Build history of the part. All positions in model axes, mm. Give positions to 0.01 mm unless a question says otherwise; leave off trailing zeros. Order: outer loops, then holes, each group sorted by start corner. A loop starts at its lowest first (then second) coordinate and runs counter-clockwise, first axis right, second up. Notation, with made-up numbers: M 34.25,-19.75 L 52.25,-19.75 A8 ccw 52.25,-11.75 Z; hole C 51.25,-8.5 d6. An arc over 180 degrees is marked long. Use CSV: the item, a comma, the result in double quotes. Start each with the question number.
Item 1: Wall check: line 1 along X through (y, z) = (29.5, -5); line 2 along Y through (x, z) = (41, -1.5); line 3 along X through (y, z) = (-29, -12.5). Give the ranges that are in metal, low to high.
Item 2: Band-saw the part on A-A on x = 0. Write the cut outline in (y, z), plus the area to 3 significant figures.
Item 3: Band-saw the part on D-D on x = -36.5. Write the cut outline in (y, z), plus the area to 3 significant figures.
Item 4: Band-saw the part on B-B on y = 0. Write the cut outline in (x, z).
Item 5: Pin check, flat tip, straight feed: P1, Ø4, axis at y = 32.5, z = -12, coming from the +X side. Stop position of the tip, or through.
Item 6: Band-saw the part on C-C on z = -11. Write the cut outline in (x, y) (3 decimals), plus the area to 3 significant figures.
Item 7: Two-plate mould, pull along Y, no slides. Class faces 1 (the cylindrical face through (33.874, -27.927, -7.888)), 2 (the flat face through (-1, 42, -10)), 3 (the flat face through (-52, 0, -10)): pulls with the +Y half, pulls with the -Y half, needs draft (parallel to the pull), parting line crosses it, or undercut.
from build123d import *

# Parameters (mm, degrees)
F0_W     = 104
F0_H     = 84
F1_DEPTH = 16
F3_R     = 4.5
F4_DEPTH = 25
F5_R     = 27
F6_DEPTH = 25
F7_R     = 13
F8_R     = 5


with BuildPart() as f1:
    # F0 (on Top) → F1 (new body)
    with BuildSketch(Plane.XY):
        Rectangle(F0_W, F0_H)
    extrude(amount=-F1_DEPTH)

    # F3 (on face) → F4 (cut)
    with BuildSketch(Plane.XY):
        with Locations((38.36957, 28.125)):
            Circle(F3_R)
        with Locations((38.36957, -28.125)):
            Circle(F3_R)
        with Locations((-38.36957, 28.125)):
            Circle(F3_R)
        with Locations((-38.36957, -28.125)):
            Circle(F3_R)
    extrude(amount=-F4_DEPTH, mode=Mode.SUBTRACT)

    # F5 (on Top) → F6 (cut)
    with BuildSketch(Plane.XY):
        Circle(F5_R)
    extrude(amount=-F6_DEPTH, mode=Mode.SUBTRACT)

    # F7
    f7_edges = [f1.edges().sort_by_distance(p)[0] for p in [
        (-52, 42, -8),
        (-52, -42, -8),
        (52, -42, -8),
        (52, 42, -8),
    ]]
    fillet(f7_edges, radius=F7_R)

    # F8
    f8_edges = [f1.edges().sort_by_distance(p)[0] for p in [
        (-52, 0, 0),
    ]]
    fillet(f8_edges, radius=F8_R)


solid = f1.part
Model answer:
1,line 1,"x = -51.99 to -42.65, -34.08 to 34.08, 42.65 to 51.99"
1,line 2,"y = -40.4 to -31.78, -24.47 to 24.47, 31.78 to 40.4"
1,line 3,"x = -52 to -42.78, -33.96 to 33.96, 42.78 to 52"
2,outline,"M -42,-16 L -27,-16 L -27,0 L -37,0 A5 ccw -42,-5 Z; M 27,-16 L 42,-16 L 42,-5 A5 ccw 37,0 L 27,0 Z"
2,area,"469 mm^2"
3,outline,"M -42,-16 L -32.22,-16 L -32.22,0 L -37,0 A5 ccw -42,-5 Z; M -24.03,-16 L 24.03,-16 L 24.03,0 L -24.03,0 Z; M 32.22,-16 L 42,-16 L 42,-5 A5 ccw 37,0 L 32.22,0 Z"
3,area,"1,070 mm^2"
4,outline,"M -52,-16 L -27,-16 L -27,0 L -47,0 A5 ccw -52,-5 Z; M 27,-16 L 52,-16 L 52,-5 A5 ccw 47,0 L 27,0 Z"
5,P1,"stops at x = 51.91"
6,outline,"M -52,-29 A13 ccw -39,-42 L 39,-42 A13 ccw 52,-29 L 52,29 A13 ccw 39,42 L -39,42 A13 ccw -52,29 Z; hole C -38.37,-28.125 d9; hole C -38.37,28.125 d9; hole C 0,0 d54; hole C 38.37,-28.125 d9; hole C 38.37,28.125 d9"
6,area,"6,050 mm^2"
7,face 1,"undercut"
7,face 2,"pulls with the +Y half"
7,face 3,"needs draft"
